from build123d import *

# Parameters (mm, degrees)
SKETCH2_R          = 30
CUT_EXTRUDE1_DEPTH = 278.128129211


with BuildPart() as part:
    # Sketch1 → Revolve1 (revolve)
    with BuildSketch(Plane.XY, mode=Mode.PRIVATE) as revolve1_sk:
        Polygon((0, 0), (0, 67.475728155), (10, 67.475728155), (10, 160), (30, 160), (30, 130), (67, 130), (80, 117), (93, 130), (130, 130), (130, 160), (150, 160), (150, 67.475728155), (160, 67.475728155), (160, 0), align=None)
    revolve(revolve1_sk.sketch.rotate(Axis((0, 0, 0), (1, 0, 0)), 90), axis=Axis((0, 0, 0), (1, 0, 0)))

    # Sketch2 → Cut-Extrude1 (cut, through all)
    with BuildSketch(Plane(origin=(160, 0, 0), x_dir=(0, 0, -1), z_dir=(1, 0, 0))):
        Circle(SKETCH2_R)
    extrude(amount=-CUT_EXTRUDE1_DEPTH, mode=Mode.SUBTRACT)


solid = part.part
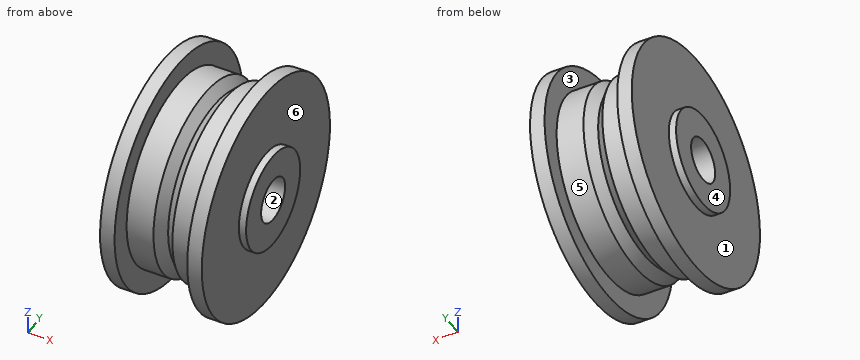
Geometry: final body of the model. Coordinates: model frame, mm. Face numbers are marked on the shaded views. A direction names the side the tool comes from. Round coordinates to 2 decimals unless told otherwise and drop trailing zeros. Order: outer loops, then holes, each group sorted by start corner. A loop starts at its lowest first (then second) coordinate and runs counter-clockwise, first axis right, second up. Notation, with made-up numbers: (15, -22.75) - (61, -22.75) arc R9 cw to (61, -13.75) - close; hole circle Ø1 at (48, 31). An arc over 180 degrees is marked (long way). Write each question's results on one line, items separated by ' | '.
Item 1: Material intervals for line 1 along X through (y, z) = (-123, -93); line 2 along Y through (x, z) = (64, 0); line 3 along Y through (x, z) = (69, 0), sorted ascending. Write a range as [from, to].
Completed:
line 1: [10, 30], [130, 150] | line 2: [-130, -30], [30, 130] | line 3: [-128, -30], [30, 128]
Item 2: Mould query, pull axis X, two halves, no side actions, for the marked faces 1, 2 and 3. Classes: pulls with the +X half, pulls with the -X half, needs draft (parallel to the pull), parting line crosses it, or undercut.
Completed:
face 1: pulls with the -X half | face 2: needs draft | face 3: undercut
Item 3: Reachability of the marked faces 4, 5 and 6 from +Z, -Z, +X, -X, +Y, -Y: full face, straight path, thin tool, end or side. Return the list, or none.
Completed:
face 4: +Z, -Z, -X, +Y, -Y | face 5: none | face 6: +X
Item 4: Section C-C, the plane x = 84. Return the cut outline in (y, z), and give its area (3 significant figures).
Completed:
outline: circle Ø242 at (0, 0); hole circle Ø60 at (0, 0) | area: 43,200 mm^2
Item 5: First-contact query: pin 1 Ø6 at (y, z) = (-110, -45.5) entering from +X; pin 2 Ø8 at (x, z) = (66.5, -37) entering from +Y; pin 3 Ø4 at (x, y) = (18.5, -73) entering from +Z. Flat tips, straight axial feed; report the tip coordinate or a pass-through.
Completed:
pin 1: x = 150 | pin 2: y = 125.74 | pin 3: z = 143.38
Item 6: Section D-D, the plane z = 137.5. Return the cut outline in (x, y), and give its area (3 significant figures).
Completed:
outline: (10, -81.82) - (30, -81.82) - (30, 81.82) - (10, 81.82) - close; (130, -81.82) - (150, -81.82) - (150, 81.82) - (130, 81.82) - close | area: 6,550 mm^2
